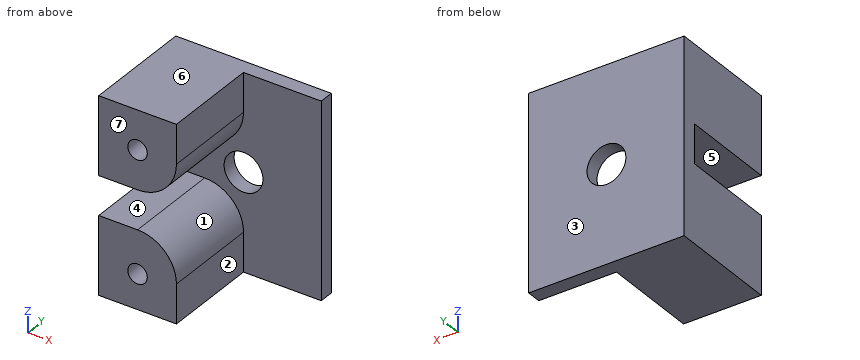
```python
from build123d import *

# Parameters (mm, degrees)
F0_W        = 101.6
F0_H        = 127
F1_DEPTH    = 9.525
F2_R        = 12.7
F3_DEPTH    = 63.5
F4_W        = 50.8
F4_H        = 50.8
F5_DEPTH    = 63.5
F6_W        = 50.8
F6_H        = 50.8
F7_DEPTH    = 63.5
F8_T1_DEPTH = 127
F9_R        = 25.4
F10_R       = 6.35
F11_DEPTH   = 12.7
F12_R       = 6.35
F13_DEPTH   = 12.7


# Not quite as in the source:
# - a fillet or chamfer that OpenCascade refuses, or shapes differently, is made with other operations: its cross-section is extruded or revolved along the edge and cut away or added


with BuildPart() as f1:
    # F0 (on Front) → F1 (new body)
    with BuildSketch(Plane.XZ):
        Rectangle(F0_W, F0_H)
    extrude(amount=F1_DEPTH)

    # F2 (on face) → F3 (cut)
    with BuildSketch(Plane.XZ.offset(9.525)):
        Circle(F2_R)
    extrude(amount=-F3_DEPTH, mode=Mode.SUBTRACT)

    # F4 (on face) → F5 (join)
    with BuildSketch(Plane.XZ.offset(9.525)):
        with Locations((-25.4, -38.1)):
            Rectangle(F4_W, F4_H)
    extrude(amount=F5_DEPTH)

    # F6 (on face) → F7 (join)
    with BuildSketch(Plane.XZ.offset(9.525)):
        with Locations((-25.4, 38.1)):
            Rectangle(F6_W, F6_H)
    extrude(amount=F7_DEPTH)

    # F8: fillet of radius 25.4 on 1 edges, made by hand

    # F8_s2 → F8_t1 (cut)
    with BuildSketch(Plane.XZ.offset(9.525)):
        with BuildLine():
            ThreePointArc((-25.4, -12.7), (-7.4394877579, -20.1394877579), (0, -38.1))
            Line((0, -38.1), (0, -12.7))
            Line((0, -12.7), (-25.4, -12.7))
        make_face()
    extrude(amount=F8_T1_DEPTH, mode=Mode.SUBTRACT)

    # F9
    f9_edges = [f1.edges().sort_by_distance(p)[0] for p in [
        (0, -41.275, 12.7),
    ]]
    fillet(f9_edges, radius=F9_R)

    # F10 (on face) → F11 (cut)
    with BuildSketch(Plane.XZ.offset(73.025)):
        with Locations((-25.4, -40.7783836126)):
            Circle(F10_R)
    extrude(amount=-F11_DEPTH, mode=Mode.SUBTRACT)

    # F12 (on face) → F13 (cut)
    with BuildSketch(Plane.XZ.offset(73.025)):
        with Locations((-25.4, 38.1)):
            Circle(F12_R)
    extrude(amount=-F13_DEPTH, mode=Mode.SUBTRACT)


solid = f1.part
```
Input: part model. Units: mm. Frame: model coordinates. Face numbers are marked on the shaded views. A direction names the side the tool comes from. Round coordinates to 2 decimals unless told otherwise and drop trailing zeros. Loops run counter-clockwise (first coordinate to the right, second up) from the corner with the lowest first, then second, coordinate; pieces in that order, holes last. Notation, with made-up numbers: (55, -26.5) - (112, -26.5) arc R13 cw to (112, -4.5) - close; hole circle Ø10 at (-38.75, 25.5). An arc over 180 degrees is marked (long way). One line per item, written item: value. Start each with the question number.
(1) Draft query along Z for the marked faces 4, 5, 6 and 7. Return one class per face: +Z half, -Z half, draft (parallel to the pull), parting line (faces both ways), or undercut.
(2) Section C-C, the plane y = -67.5. Return loops of the section in (x, z), plus the area to 3 significant figures.
(3) Section A-A, the plane z = 0. Return loops of the section in (x, y) (3 decimals), plus the area to 3 significant figures.
(4) Section D-D, the plane x = -7.5. Return loops of the section in (y, z) (3 decimals), plus the area to 3 significant figures.
(5) Contact query for flat-ended pins moving along their axis: P1, Ø4, axis at x = -28, z = 39.5, coming from the -Y side (3 decimals); P2, Ø4, axis at x = 3.5, y = -33.5, coming from the +Z side; P3, Ø3, axis at x = 28.5, z = -44, coming from the -Y side (3 decimals); P4, Ø20.5, axis at y = -28.5, z = -55.5, coming from the +X side. Output: stop coordinate, or through.
(6) Access query for the marked faces 1, 2 and 3. Directions: +Z, -Z, +X, -X, +Y, -Y. A direction counts if a zero-diameter tool reaches every point of the face in a straight line with its end or side. Return the directions, or none.
(7) Section B-B, the plane y = -36. Return loops of the section in (x, z), plus the area to 3 significant figures.
(8) Ray query, line 1 (Z direction, x = -25, y = -70); line 2 (X direction, y = -3.5, z = 0); line 3 (X direction, y = -69, z = 38). Return the intervals inside material, ascending. Write a range as [from, to].
Results below:
1. face 4: undercut
1. face 5: undercut
1. face 6: +Z half
1. face 7: draft
2. outline: (-50.8, -63.5) - (0, -63.5) - (0, -38.1) arc R25.4 ccw to (-25.4, -12.7) - (-50.8, -12.7) - close; (-50.8, 12.7) - (-25.4, 12.7) arc R25.4 ccw to (0, 38.1) - (0, 63.5) - (-50.8, 63.5) - close; hole circle Ø12.7 at (-25.4, -40.78); hole circle Ø12.7 at (-25.4, 38.1)
2. area: 4,630 mm^2
3. outline: (-50.8, -9.525) - (-12.7, -9.525) - (-12.7, 0) - (-50.8, 0) - close; (12.7, -9.525) - (50.8, -9.525) - (50.8, 0) - (12.7, 0) - close
3. area: 726 mm^2
4. outline: (-73.025, -63.5) - (0, -63.5) - (0, -10.249) - (-9.525, -10.249) - (-9.525, -20.079) - (-73.025, -20.079) - close; (-73.025, 20.079) - (-9.525, 20.079) - (-9.525, 10.249) - (0, 10.249) - (0, 63.5) - (-73.025, 63.5) - close
4. area: 6,530 mm^2
5. P1: y = -60.325
5. P2: through
5. P3: y = -9.525
5. P4: x = 0
6. face 1: +X, -Y
6. face 2: +Z, -Z, +X, -Y
6. face 3: +Z, -Z, +X, -X, +Y
7. outline: (-50.8, -63.5) - (0, -63.5) - (0, -38.1) arc R25.4 ccw to (-25.4, -12.7) - (-50.8, -12.7) - close; (-50.8, 12.7) - (-25.4, 12.7) arc R25.4 ccw to (0, 38.1) - (0, 63.5) - (-50.8, 63.5) - close
7. area: 4,880 mm^2
8. line 1: [-63.5, -47.12], [-34.44, -12.7], [12.7, 31.76], [44.44, 63.5]
8. line 2: [-50.8, -12.7], [12.7, 50.8]
8. line 3: [-50.8, -31.75], [-19.05, 0]
